Source: three-view drawing plus pictorial views. Frame: mm from the lowest corner of the part. A direction names the side the tool comes from. Give positions to 0.01 mm unless a question says otherwise; leave off trailing zeros. Order: outer loops, then holes, each group sorted by start corner. A loop starts at its lowest first (then second) coordinate and runs counter-clockwise, first axis right, second up.
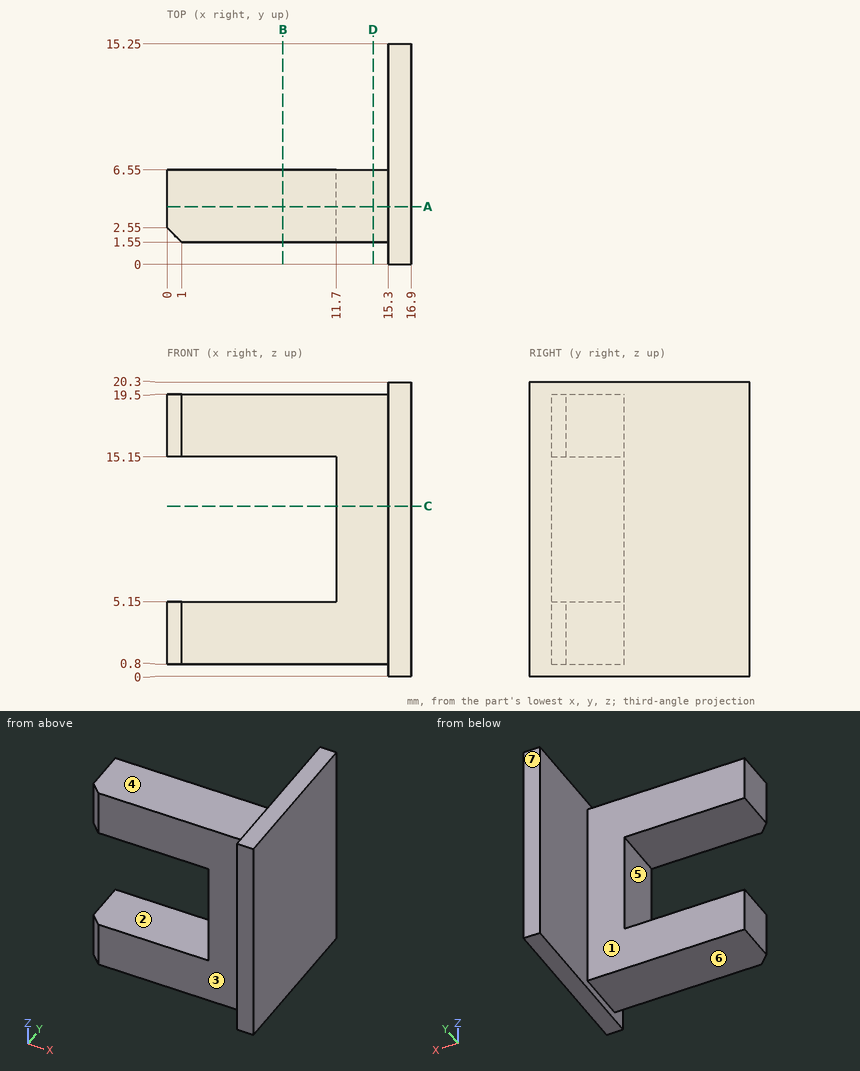
1) Ray query, L1, parallel to Z at x = 11, y = 3.25; L2, parallel to X at y = 8, z = 2.5; L3, parallel to Z at x = 12.25, y = 6.5. Return the intervals inside material, ascending.
Checks:
L1: z = 0.8 to 5.15, 15.15 to 19.5
L2: x = 15.3 to 16.9
L3: z = 0.8 to 19.5
2) Reachability of the marked faces 1, 2 and 3 from +Z, -Z, +X, -X, +Y, -Y: full face, straight path, thin tool, end or side. Return the list, or none.
Checks:
face 1: +Z, -Z, -X, +Y
face 2: -X, +Y, -Y
face 3: +Z, -Z, -X, -Y
3) Section query B-B on x = 8. Output: boundary loops of the cut face in (y, z).
Checks:
outline: (1.55, 0.8) - (6.55, 0.8) - (6.55, 5.15) - (1.55, 5.15) - close; (1.55, 15.15) - (6.55, 15.15) - (6.55, 19.5) - (1.55, 19.5) - close
4) Section query C-C on z = 11.75. Output: boundary loops of the cut face in (x, y), and give its area (3 significant figures).
Checks:
outline: (11.7, 1.55) - (15.3, 1.55) - (15.3, 0) - (16.9, 0) - (16.9, 15.25) - (15.3, 15.25) - (15.3, 6.55) - (11.7, 6.55) - close
area: 42.4 mm2
5) First-contact query: pin 1 Ø4.5 at (y, z) = (10.5, 12) entering from -X; pin 2 Ø1.5 at (y, z) = (1.5, 16) entering from -X; pin 3 Ø4.5 at (x, z) = (7.5, 13.5) entering from +Y. Flat tips, straight axial feed; report the tip coordinate or a pass-through.
Checks:
pin 1: stops at x = 15.3
pin 2: stops at x = 0.3
pin 3: stops at y = 6.55
6) Pull-direction query (Z, two-part tool) for the marked faces 4, 5, 6 and 7; classes: +Z half, -Z half, draft (parallel to the pull), parting line (faces both ways), or undercut.
Checks:
face 4: +Z half
face 5: undercut
face 6: -Z half
face 7: draft
7) Section query A-A on y = 4. Output: boundary loops of the cut face in (x, z), and give its area (3 significant figures).
Checks:
outline: (0, 0.8) - (15.3, 0.8) - (15.3, 0) - (16.9, 0) - (16.9, 20.3) - (15.3, 20.3) - (15.3, 19.5) - (0, 19.5) - (0, 15.15) - (11.7, 15.15) - (11.7, 5.15) - (0, 5.15) - close
area: 202 mm2
8) Section query D-D on x = 14.25. Output: boundary loops of the cut face in (y, z), and give its area (3 significant figures).
Checks:
outline: (1.55, 0.8) - (6.55, 0.8) - (6.55, 19.5) - (1.55, 19.5) - close
area: 93.5 mm2
